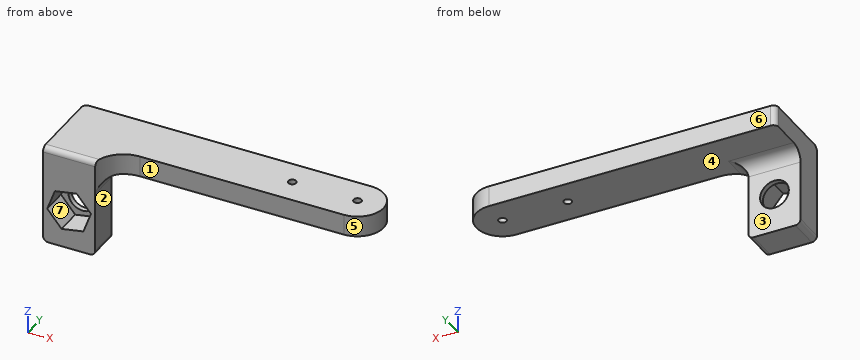
from build123d import *

# Parameters (mm, degrees)
BOSS_EXTRUDE1_DEPTH      = 8
SKETCH2_R                = 1.5
CUT_EXTRUDE1_DEPTH       = 10
BOSS_EXTRUDE3_DEPTH      = 30
BOSS_EXTRUDE3_DEPTH_BACK = 8
SKETCH6_W                = 20
SKETCH6_H                = 10
FILLET3_R                = 12
SKETCH7_W                = 20
SKETCH7_H                = 30
BOSS_EXTRUDE4_DEPTH      = 2
CUT_EXTRUDE3_DEPTH       = 10
SKETCH9_R                = 5.5
CUT_EXTRUDE4_DEPTH       = 10
FILLET4_R                = 5
FILLET5_R                = 2
SKETCH10_R               = 1.5
CUT_EXTRUDE5_DEPTH       = 10


with BuildPart() as part:
    # Sketch1 → Boss-Extrude1 (new body)
    with BuildSketch(Plane.XY):
        with BuildLine():
            Line((-25, 10), (85, 10))
            ThreePointArc((85, 10), (95, 0), (85, -10))
            Line((85, -10), (-25, -10))
            Line((-25, -10), (-25, 10))
        make_face()
    extrude(amount=BOSS_EXTRUDE1_DEPTH)

    # Sketch2 → Cut-Extrude1 (cut)
    with BuildSketch(Plane.XY.offset(8)):
        with Locations((85, 0)):
            Circle(SKETCH2_R)
    extrude(amount=-CUT_EXTRUDE1_DEPTH, mode=Mode.SUBTRACT)

    # Sketch6 → Boss-Extrude3 (add, two sides: drawn at the far end of the back side and taken through both)
    with BuildSketch(Plane(origin=(0, 0, 0), x_dir=(-1, 0, 0), z_dir=(0, 0, -1)).offset(-BOSS_EXTRUDE3_DEPTH_BACK)):
        with Locations((15, -15)):
            Rectangle(SKETCH6_W, SKETCH6_H)
    extrude(amount=BOSS_EXTRUDE3_DEPTH + BOSS_EXTRUDE3_DEPTH_BACK)

    # Fillet3
    # the kernel refuses this fillet: 12 mm, written as the material it adds along each edge
    with BuildSketch(Plane(origin=(-5, -10, 8), x_dir=(0, -1, 0), z_dir=(0, 0, -1))) as fillet3_piece_1:
        with BuildLine():
            CenterArc((12, -11.832159566), FILLET3_R, 99.594068227, 80.405931773)
            Line((0, -11.832159566), (0, 0))
            Line((0, 0), (10, 0))
        make_face()
    extrude(amount=8)

    # Sketch7 → Boss-Extrude4 (add)
    with BuildSketch(Plane(origin=(0, -10, 0), x_dir=(1, 0, 0), z_dir=(0, 1, 0))):
        with Locations((-15, 15)):
            Rectangle(SKETCH7_W, SKETCH7_H)
    extrude(amount=BOSS_EXTRUDE4_DEPTH)

    # Sketch8 → Cut-Extrude3 (cut)
    with BuildSketch(Plane.XZ.offset(20)):
        Polygon((-12.092828782, -7.012612723), (-20.463694682, -8.488622233), (-23.370865901, -16.47600951), (-17.907171218, -22.987387277), (-9.536305318, -21.511377767), (-6.629134099, -13.52399049), align=None)
    extrude(amount=-CUT_EXTRUDE3_DEPTH, mode=Mode.SUBTRACT)

    # Sketch9 → Cut-Extrude4 (cut)
    with BuildSketch(Plane.XZ.offset(10)):
        with Locations(Location((-15, -15, 0), (0, 0, 270))):
            Circle(SKETCH9_R)
    extrude(amount=-CUT_EXTRUDE4_DEPTH, mode=Mode.SUBTRACT)

    # Fillet4
    # the kernel refuses this fillet: 5 mm, written as the material it adds along each edge
    with BuildSketch(Plane(origin=(-5, -20, 0), x_dir=(1, 0, 0), z_dir=(0, 1, 0))) as fillet4_piece_1_section:
        with BuildLine():
            CenterArc((FILLET4_R, FILLET4_R), FILLET4_R, 180, 90)
            Line((0, FILLET4_R), (0, 0))
            Line((0, 0), (FILLET4_R, 0))
        make_face()
    fillet4_piece_1 = extrude(amount=12, mode=Mode.PRIVATE)
    fillet4_piece_1 = fillet4_piece_1 - Plane(origin=(6.832159566, -22, 0), x_dir=(0, -1, 0), z_dir=(0, 0, 1)) * Cylinder(12, 44, mode=Mode.PRIVATE)
    add(fillet4_piece_1)
    with BuildSketch(Plane(origin=(-25, -8, 0), x_dir=(0, 1, 0), z_dir=(1, 0, 0))) as fillet4_piece_2:
        with BuildLine():
            CenterArc((FILLET4_R, -FILLET4_R), FILLET4_R, 90, 90)
            Line((0, -FILLET4_R), (0, 0))
            Line((0, 0), (FILLET4_R, 0))
        make_face()
    extrude(amount=20)
    with BuildSketch(Plane(origin=(-5, -20, 0), x_dir=(1, 0, 0), z_dir=(0, 1, 0))) as fillet4_piece_3a_section:
        with BuildLine():
            CenterArc((FILLET4_R, FILLET4_R), FILLET4_R, 180, 90)
            Line((0, FILLET4_R), (0, 0))
            Line((0, 0), (FILLET4_R, 0))
        make_face()
    fillet4_piece_3a = extrude(amount=24.5, mode=Mode.PRIVATE)
    fillet4_piece_3a = split(fillet4_piece_3a, bisect_by=Plane(origin=(-5, -8, 0), z_dir=(0, 1, 0)), keep=Keep.TOP, mode=Mode.PRIVATE)
    with BuildSketch(Plane(origin=(-25, -8, 0), x_dir=(0, 1, 0), z_dir=(1, 0, 0))) as fillet4_piece_3b_section:
        with BuildLine():
            CenterArc((FILLET4_R, -FILLET4_R), FILLET4_R, 90, 90)
            Line((0, -FILLET4_R), (0, 0))
            Line((0, 0), (FILLET4_R, 0))
        make_face()
    fillet4_piece_3b = extrude(amount=32.5, mode=Mode.PRIVATE)
    fillet4_piece_3b = split(fillet4_piece_3b, bisect_by=Plane(origin=(-5, -8, 0), z_dir=(1, 0, 0)), keep=Keep.TOP, mode=Mode.PRIVATE)
    fillet4_piece_3 = fillet4_piece_3a & fillet4_piece_3b
    add(fillet4_piece_3)

    # Fillet5
    fillet5_edges = [part.edges().sort_by_distance(p)[0] for p in [
        (-15, -20, 8),
        (-25, -14, -30),
        (-5, -14, -30),
        (-25, 10, 4),
    ]]
    fillet(fillet5_edges, radius=FILLET5_R)

    # Sketch10 → Cut-Extrude5 (cut)
    with BuildSketch(Plane.XY.offset(8)):
        with Locations((60, 0)):
            Circle(SKETCH10_R)
    extrude(amount=-CUT_EXTRUDE5_DEPTH, mode=Mode.SUBTRACT)


solid = part.part
Verification items for the finished model (mm, model axes). Face numbers are marked on the shaded views. A direction names the side the tool comes from. Coordinates: 2 decimals unless noted, no trailing zeros. Loops run counter-clockwise (first coordinate to the right, second up) from the corner with the lowest first, then second, coordinate; pieces in that order, holes last. Notation, with made-up numbers: (8.5, 31) -> (51.5, 31) arc R23 ccw to (51.5, 45) -> close; hole circle Ø8 at (82, 11.5). An arc over 180 degrees is marked (long way). Write each question's results on one line, items separated by ' | '.
Item 1: Section check A-A, the plane x = 60. Enter the section's corners in (y, z), plus the area to 3 significant figures.
Found:
outline: (-10, 0) -> (-1.5, 0) -> (-1.5, 8) -> (-10, 8) -> close; (1.5, 0) -> (10, 0) -> (10, 8) -> (1.5, 8) -> close | area: 136 mm2
Item 2: Material ranges on L1, parallel to X at y = -8.35, z = -15; L2, parallel to Y at x = 85, z = 5; L3, parallel to Z at x = 73, y = -6.5, recorded low to high.
Found:
L1: x = -25 to -20.5, -9.5 to -5 | L2: y = -10 to -1.5, 1.5 to 10 | L3: z = 0 to 8
Item 3: Tool access check on the marked faces 1, 2, 3 and 4. Record the directions out of +Z, -Z, +X, -X, +Y, -Y that give a thin tool (end or side, any length) a straight path to the whole face; none if there is none.
Found:
face 1: +Z, -Z, +X, -Y | face 2: -Z, +X, +Y, -Y | face 3: -Z, +X, -X, +Y | face 4: -Z, +X, +Y
Item 4: Section check D-D, the plane y = -16.5. Enter the section's corners in (x, z).
Found:
outline: (-25, -28) arc R2 ccw to (-23, -30) -> (-7, -30) arc R2 ccw to (-5, -28) -> (-5, -5) arc R5 cw to (-3.83, -1.79) -> (-3.83, 8) -> (-25, 8) -> close; hole (-23.37, -16.48) -> (-17.91, -22.99) -> (-9.54, -21.51) -> (-6.63, -13.52) -> (-12.09, -7.01) -> (-20.46, -8.49) -> close
Item 5: Section check B-B, the plane y = 0. Enter the section's corners in (x, z), plus the area to 3 significant figures.
Found:
outline: (-25, 0) -> (58.5, 0) -> (58.5, 8) -> (-25, 8) -> close; (61.5, 0) -> (83.5, 0) -> (83.5, 8) -> (61.5, 8) -> close; (86.5, 0) -> (95, 0) -> (95, 8) -> (86.5, 8) -> close | area: 912 mm2
Item 6: Mould release check, pull along X, two halves, no side actions. Record for the marked faces 5, 6 and 7: +X half, -X half, draft (parallel to the pull), parting line (faces both ways), or undercut.
Found:
face 5: +X half | face 6: draft | face 7: undercut
Item 7: Gauge pin test, flat ends, axial feed: pin 1 (22 mm diameter, centred on x = -11, z = -14.5, fed in from +Y); pin 2 (3.5 mm diameter, centred on y = -17, z = -11, fed in from +X); pin 3 (6.5 mm diameter, centred on x = 51, z = 5.5, fed in from -Y). Record the tip position at first contact, or that the pin passes through.
Found:
pin 1: stops at y = -7.77 | pin 2: stops at x = -5 | pin 3: stops at y = -10
Item 8: Section check C-C, the plane z = -15. Enter the section's corners in (x, y), plus the area to 3 significant figures.
Found:
outline: (-25, -20) -> (-22.83, -20) -> (-22.83, -10) -> (-20.5, -10) -> (-20.5, -8) -> (-25, -8) -> close; (-9.5, -10) -> (-7.17, -10) -> (-7.17, -20) -> (-5, -20) -> (-5, -8) -> (-9.5, -8) -> close | area: 61.3 mm2
